Autodesk Inventor part; units mm, degrees
ref_plane "YZ Plane" through (0, 0, 0) normal (1, 0, 0) x (0, 1, 0)
ref_plane "XY Plane" through (0, 0, 0) normal (0, 0, 1) x (1, 0, 0)
sketch "Sketch1" plane through (0, 0, 0) normal (0, 1, 0) x (-1, 0, 0)
  circle A0 centre (0, 0) radius 10
  circle A1 centre (0, 0) radius 11.5
  dimension "d0" = 20
  dimension "d1" = 23
extrude "Extrusion1" add sketch "Sketch1" along normal blind 40
sketch "Sketch2" plane through (0, 40, 0) normal (0, 1, 0) x (1, 0, 0)
  circle A0 centre (0, 0) radius 9.75
  circle A1 centre (0, 0) radius 9
  dimension "d4" = 19.5
extrude "Extrusion2" add sketch "Sketch2" along normal blind 35
sketch "Sketch3" plane through (0, 40, 0) normal (0, 1, 0) x (1, 0, 0)
  circle A0 centre (0, 0) radius 9.75
  circle A1 centre (0, 0) radius 11.5
extrude "Extrusion3" add sketch "Sketch3" along normal blind 5
fillet "Fillet1" radius 5 2 edges at (-9.75, 45, 0) (-11.5, 45, 0)
fillet "Fillet2" radius 5 2 edges at (-9, 40, 0) (10, 40, 0)
ref_plane "Work Plane1" through (0, 50, 0) normal (0, 1, 0) x (-1, 0, 0)
sketch "Sketch4" plane through (0, 50, 0) normal (0, 1, 0) x (-1, 0, 0)
  circle A0 centre (0, 0) radius 11.5
  line L0 (0, -11.5) -> (38, -11.5)
  line L1 (40, -9.5) -> (40, 9.5)
  line L2 (38, 11.5) -> (0, 11.5)
  arc A1 (40, 9.5) -> (38, 11.5) centre (38, 9.5) ccw
  arc A2 (38, -11.5) -> (40, -9.5) centre (38, -9.5) ccw
  circle A3 centre (0, 0) radius 9.75
  spline S0 degree 2 poles (0, -11.5) (-3.8325, -11.5) (-6, -7.6852) knots 0 0 0 1 1 1
  spline S1 degree 2 poles (0, 11.5) (-3.8325, 11.5) (-6, 7.6852) knots 0 0 0 1 1 1
  point P0 (40, -11.5)
  dimension "d19" = 40
  dimension "d20" = 2
extrude "Extrusion5" add sketch "Sketch4" along normal blind 5 contours A0 S0 A3 S1 | A0 L2 A1 L1 A2 L0 picked at (10.8206, -0.853)
properties part number "Elbow Extension"
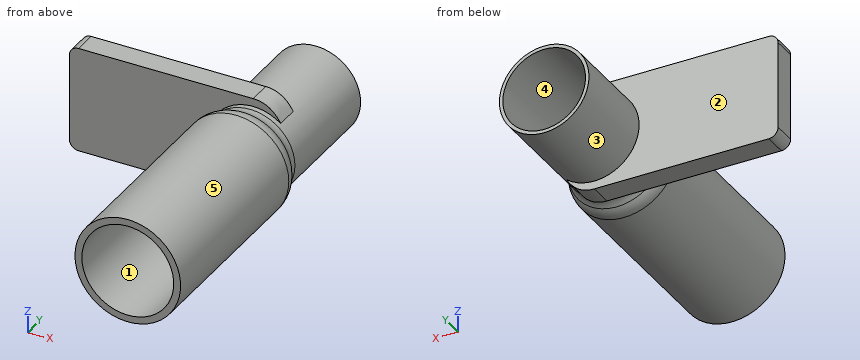
Verification items for the finished model (mm, model axes). Face numbers are marked on the shaded views. A direction names the side the tool comes from. Round coordinates to 2 decimals unless told otherwise and drop trailing zeros. Loops run counter-clockwise (first coordinate to the right, second up) from the corner with the lowest first, then second, coordinate; pieces in that order, holes last. Notation, with made-up numbers: (45, 74.25) - (80, 74.25) arc R23 ccw to (80, 96.25) - close; hole circle Ø1 at (72, 70). An arc over 180 degrees is marked (long way). Use a Markdown table: item, result. Add a question column.
1. Section check C-C, the plane y = 13. Record the boundary of the cut face in (x, z).
2. Access from +Z, -Z, +X, -X, +Y, -Y to the whole of each face (thin tool, end or side, straight path). Record for the marked faces 4 and 5.
3. Release check for a two-part mould opening along Z. For the marked faces 1, 2 and 3 record: released by +Z, released by -Z, zero draft, split by the parting line, or undercut.
4. Gauge pin test, flat ends, axial feed: pin 1 (1 mm diameter, centred on y = 47.5, z = -6.5, fed in from +X); pin 2 (1 mm diameter, centred on x = -7, y = 22, fed in from -Z); pin 3 (1 mm diameter, centred on y = 48.5, z = 5, fed in from +X); pin 4 (11 mm diameter, centred on x = 0, z = 0, fed in from -Y). Record the tip position at first contact, or that the pin passes through.
5. Section check B-B, the plane x = -19. Record the boundary of the cut face in (y, z), plus the area to 3 significant figures.
6. Thickness scan on probe 1 along Z at (x, y) = (0, 53); probe 2 along Z at (x, y) = (0, 62); probe 3 along Y at (x, z) = (-24, -1.25). Record the ranges inside material, lowest first. Write a range as [from, to].
7. Section check A-A, the plane y = 57. Record the boundary of the cut face in (x, z), plus the area to 3 significant figures.
Checks:
| question | item | result |
|---|---|---|
| 1 | outline | circle Ø23 at (0, 0); hole circle Ø20 at (0, 0) |
| 2 | face 4 | +Y, -Y |
| 2 | face 5 | -Y |
| 3 | face 1 | undercut |
| 3 | face 2 | zero draft |
| 3 | face 3 | split by the parting line |
| 4 | pin 1 | stops at x = 7.94 |
| 4 | pin 2 | stops at z = -9.49 |
| 4 | pin 3 | stops at x = 8.66 |
| 4 | pin 4 | passes through |
| 5 | outline | (50, -11.5) - (55, -11.5) - (55, 11.5) - (50, 11.5) - close |
| 5 | area | 115 mm^2 |
| 6 | probe 1 | z = [-11.5, -9], [9, 11.5] |
| 6 | probe 2 | z = [-9.75, -9], [9, 9.75] |
| 6 | probe 3 | y = [50, 55] |
| 7 | outline | circle Ø19.5 at (0, 0); hole circle Ø18 at (0, 0) |
| 7 | area | 44.2 mm^2 |
